Geometry: final body of the model. Coordinates: model frame, mm. Give positions to 0.01 mm unless a question says otherwise; leave off trailing zeros. Write each loop counter-clockwise with the first axis right and the second up, starting at its lowest first coordinate (ties: lowest second). Pieces come first, ordered by that corner, then holes. Notation, with made-up numbers: (9, -11) -> (33, -11) arc R9 cw to (33, -3) -> close; hole circle Ø11 at (-30.5, -21). An arc over 180 degrees is marked (long way). Answer as a JSON object with one key per item and string values.
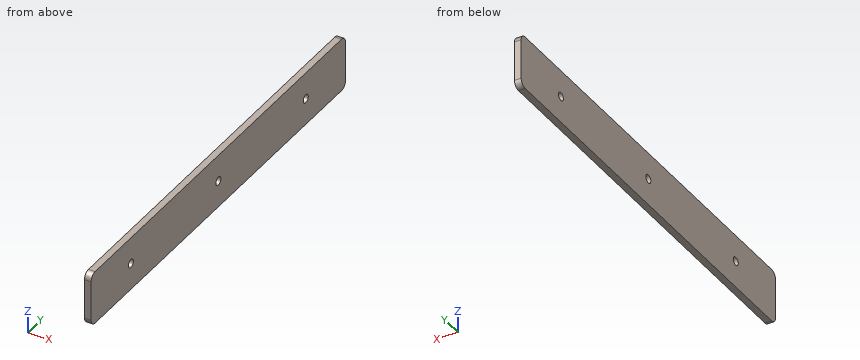
from build123d import *

# Parameters (mm, degrees)
F0_R     = 4
F1_DEPTH = 6.35


with BuildPart() as f1:
    # F0 (on Right) → F1 (new body)
    with BuildSketch(Plane.YZ):
        with BuildLine():
            ThreePointArc((203.2, 19.05), (201.340128, 23.540128), (196.85, 25.4))
            Line((196.85, 25.4), (-196.85, 25.4))
            ThreePointArc((-196.85, 25.4), (-201.340128, 23.540128), (-203.2, 19.05))
            Line((-203.2, 19.05), (-203.2, -19.05))
            ThreePointArc((-203.2, -19.05), (-201.340128, -23.540128), (-196.85, -25.4))
            Line((-196.85, -25.4), (196.85, -25.4))
            ThreePointArc((196.85, -25.4), (201.340128, -23.540128), (203.2, -19.05))
            Line((203.2, -19.05), (203.2, 19.05))
        make_face()
        with Locations((-139.7, 0)):
            Circle(F0_R, mode=Mode.SUBTRACT)
        Circle(F0_R, mode=Mode.SUBTRACT)
        with Locations((139.7, 0)):
            Circle(F0_R, mode=Mode.SUBTRACT)
    extrude(amount=F1_DEPTH)


solid = f1.part
Q1. Cut plane B-B (y = 0). Return the cut outline in (x, z).
Values:
{"outline": "(0, -25.4) -> (6.35, -25.4) -> (6.35, -4) -> (0, -4) -> close; (0, 4) -> (6.35, 4) -> (6.35, 25.4) -> (0, 25.4) -> close"}
Q2. Cut plane A-A (z = 0). Return the cut outline in (x, y).
Values:
{"outline": "(0, -203.2) -> (6.35, -203.2) -> (6.35, -143.7) -> (0, -143.7) -> close; (0, -135.7) -> (6.35, -135.7) -> (6.35, -4) -> (0, -4) -> close; (0, 4) -> (6.35, 4) -> (6.35, 135.7) -> (0, 135.7) -> close; (0, 143.7) -> (6.35, 143.7) -> (6.35, 203.2) -> (0, 203.2) -> close"}
Q3. Material intervals for L1, parallel to Z at x = 4, y = -139.7; L2, parallel to Y at x = 4.5, z = 1.5; L3, parallel to Y at x = 1.25, z = -3, sorted ascending. Write a range as from..to.
Values:
{"L1": "-25.4..-4, 4..25.4", "L2": "-203.2..-143.41, -135.99..-3.71, 3.71..135.99, 143.41..203.2", "L3": "-203.2..-142.35, -137.05..-2.65, 2.65..137.05, 142.35..203.2"}
